Autodesk Inventor part; units mm, degrees
ref_plane "YZ Plane" through (0, 0, 0) normal (1, 0, 0) x (0, 1, 0)
ref_plane "XZ Plane" through (0, 0, 0) normal (0, 1, 0) x (-1, 0, 0)
ref_plane "XY Plane" through (0, 0, 0) normal (0, 0, 1) x (1, 0, 0)
sketch "Skizze1" plane through (0, 0, 0) normal (0, 0, 1) x (1, 0, 0)
  line L0 (-14.5, 0) -> (14.5, 0)
  line L1 (14.5, 0) -> (14.5, -15)
  line L2 (-14.5, -15) -> (-14.5, 0)
  line L3 (-5.9, -15) -> (-5.9, -6.6)
  line L4 (-5.9, -6.6) -> (5.9, -6.6)
  line L5 (5.9, -6.6) -> (5.9, -15)
  line L6 (14.5, -15) -> (5.9, -15)
  line L7 (-5.9, -15) -> (-14.5, -15)
  line L8 (0, 0) -> (0, -6.6)
  line L9 (-10.2, -15) -> (-10.2, 0)
  line L10 (10.2, -15) -> (10.2, 0)
  dimension "d0" = 11.8
  dimension "d1" = 8.4
  dimension "d2" = 29
  dimension "d3" = 15
extrude "Extrusion1" add sketch "Skizze1" along normal mid plane 15
sketch "Skizze2" plane through (0, 0, 0) normal (0, 0, 1) x (1, 0, 0)
  line L0 (5.9, -15) -> (14.5, -15)
  line L1 (6.75, -15) -> (-6.75, -15)
  line L2 (-6.75, -15) -> (-6.75, -6)
  line L3 (-6.75, -6) -> (6.75, -6)
  line L4 (6.75, -6) -> (6.75, -15)
  line L5 (0, -18) -> (0, 3)
  point P0 (0, 0)
  point P1 (0, -6)
  dimension "d6" = 13.5
  dimension "d7" = 9
extrude "Extrusion2" cut sketch "Skizze2" along normal through all
sketch "Skizze3" plane through (-14.5, 0, 7.5) normal (0, 1, 0) x (1, 0, 0)
  point P0 (14.5, 7.5)
  point P1 (4.3, 7.5)
  point P2 (24.7, 7.5)
hole "Bohrung1" at (-10.2, 0, 0) at (10.2, 0, 0) direction (0, -1, 0) diameter 3 end through all counterbore diameter 6.5 counterbore depth 3.4
fillet "Rundung1" radius 0.5 26 edges at (0, 0, 7.5) (14.5, 0, 0) (0, 0, -7.5) (-14.5, 0, 0) (-6.75, -10.5, 7.5) (0, -6, 7.5) (-10.625, -15, 7.5) (-14.5, -7.5, 7.5) (6.75, -10.5, 7.5) (10.625, -15, 7.5) (14.5, -7.5, 7.5) (14.5, -7.5, -7.5) (14.5, -15, 0) (5.9, -10.8, -7.5) (0, -6.6, -7.5) (-5.9, -10.8, -7.5) (-14.5, -7.5, -7.5) (-10.2, -15, -7.5) (-5.9, -15, -3.75) (-6.75, -15, 3.75) (-14.5, -15, 0) (-6.325, -15, 0) (6.325, -15, 0) (6.75, -15, 3.75) (5.9, -15, -3.75) (10.2, -15, -7.5)
properties part number "connector_securing_V1" material "ABS-Kunststoff"
Input: part model. Units: mm. Frame: model coordinates. A direction names the side the tool comes from. Round coordinates to 2 decimals unless told otherwise and drop trailing zeros. Order: outer loops, then holes, each group sorted by start corner. A loop starts at its lowest first (then second) coordinate and runs counter-clockwise, first axis right, second up. Notation, with made-up numbers: (24, 88) - (34, 88) arc R22 ccw to (34, 121) - close; hole circle Ø6 at (6.5, -4). An arc over 180 degrees is marked (long way). Use a Markdown table: item, result.
1. Access query for faces 1 (the face through (6.75, -10, 3)), 2 (the face through (5.9, -10, -4)), 3 (the face through (-7.027, -1.724, -0.705)). Directions: +Z, -Z, +X, -X, +Y, -Y. A direction counts if a zero-diameter tool reaches every point of the face in a straight line with its end or side. Return the directions, or none.
Evaluation:
| item | result |
|---|---|
| face 1 | +Z, -Y |
| face 2 | +Z, -Z, -Y |
| face 3 | +Y |
2. Section C-C on x = 10.2. Return the cut outline in (y, z).
Evaluation:
| item | result |
|---|---|
| outline | (-15, -7) arc R0.5 ccw to (-14.5, -7.5) - (-0.5, -7.5) arc R0.5 ccw to (0, -7) - (0, -3.25) - (-3.4, -3.25) - (-3.4, -1.5) - (-15, -1.5) - close; (-15, 1.5) - (-3.4, 1.5) - (-3.4, 3.25) - (0, 3.25) - (0, 7) arc R0.5 ccw to (-0.5, 7.5) - (-14.5, 7.5) arc R0.5 ccw to (-15, 7) - close |
3. Section A-A on y = -12. Return the cut outline in (x, z), then the cut area to 3 significant figures.
Evaluation:
| item | result |
|---|---|
| outline | (-14.5, -7) arc R0.5 ccw to (-14, -7.5) - (-6.4, -7.5) arc R0.5 ccw to (-5.9, -7) - (-5.9, 0) - (-6.75, 0) - (-6.75, 7) arc R0.5 ccw to (-7.25, 7.5) - (-14, 7.5) arc R0.5 ccw to (-14.5, 7) - close; (5.9, -7) arc R0.5 ccw to (6.4, -7.5) - (14, -7.5) arc R0.5 ccw to (14.5, -7) - (14.5, 7) arc R0.5 ccw to (14, 7.5) - (7.25, 7.5) arc R0.5 ccw to (6.75, 7) - (6.75, 0) - (5.9, 0) - close; hole circle Ø3 at (-10.2, 0); hole circle Ø3 at (10.2, 0) |
| area | 231 mm^2 |
4. Mould query, pull axis Z, two halves, no side actions, for faces 4 (the face through (0, -6, 3)), 5 (the face through (-0.2, -5.8, -7.5)), 6 (the face through (11.664, -9.281, -0.325)), 7 (the face through (0, -4, 7.5)). Classes: +Z half, -Z half, draft (parallel to the pull), parting line (faces both ways), or undercut.
Evaluation:
| item | result |
|---|---|
| face 4 | draft |
| face 5 | -Z half |
| face 6 | undercut |
| face 7 | +Z half |
5. Section D-D on x = -1. Return the cut outline in (y, z), then the cut area to 3 significant figures.
Evaluation:
| item | result |
|---|---|
| outline | (-6.6, -7) arc R0.5 ccw to (-6.1, -7.5) - (-0.5, -7.5) arc R0.5 ccw to (0, -7) - (0, 7) arc R0.5 ccw to (-0.5, 7.5) - (-5.5, 7.5) arc R0.5 ccw to (-6, 7) - (-6, 0) - (-6.6, 0) - close |
| area | 94.3 mm^2 |
6. Section B-B on y = -2. Return the cut outline in (x, z).
Evaluation:
| item | result |
|---|---|
| outline | (-14.5, -7) arc R0.5 ccw to (-14, -7.5) - (14, -7.5) arc R0.5 ccw to (14.5, -7) - (14.5, 7) arc R0.5 ccw to (14, 7.5) - (-14, 7.5) arc R0.5 ccw to (-14.5, 7) - close; hole circle Ø6.5 at (-10.2, 0); hole circle Ø6.5 at (10.2, 0) |
7. Material intervals for probe 1 along X at (y, z) = (-1.85, 0); probe 2 along Z at (x, y) = (-10.2, -1.05); probe 3 along X at (y, z) = (-8.75, -4), sorted ascending.
Evaluation:
| item | result |
|---|---|
| probe 1 | -14.5 to -13.45, -6.95 to 6.95, 13.45 to 14.5 |
| probe 2 | -7.5 to -3.25, 3.25 to 7.5 |
| probe 3 | -14.5 to -5.9, 5.9 to 14.5 |
8. First-contact query: pin 1 (6 mm diameter, centred on x = 7, z = 5.5, fed in from +Y); pin 2 (5 mm diameter, centred on x = -10.2, z = 0, fed in from +Y); pin 3 (5.5 mm diameter, centred on x = -2, z = -4.5, fed in from -Y); pin 4 (4 mm diameter, centred on x = 0, y = -10, fed in from +Z). Flat tips, straight axial feed; report the tip coordinate or a pass-through.
Evaluation:
| item | result |
|---|---|
| pin 1 | y = 0 |
| pin 2 | y = -3.4 |
| pin 3 | y = -6.6 |
| pin 4 | through |
